Check sheet for the modelled part. Datum: model origin and axes. Units: mm. A direction names the side the tool comes from. Round coordinates to 2 decimals unless told otherwise and drop trailing zeros. Order: outer loops, then holes, each group sorted by start corner. A loop starts at its lowest first (then second) coordinate and runs counter-clockwise, first axis right, second up.
Q1. Cross-section at D-D on z = 5. Record the cut outline in (x, y).
Q2. Scan lines: probe 1 along Y at (x, z) = (21, 12.5); probe 2 along Y at (x, z) = (-26, 4.25); probe 3 along X at (y, z) = (21, 2). Record each from-to range of solid material in increasing order.
Q3. Cross-section at B-B on y = 32.5. Record the cut outline in (x, z), then the cut area to 3 significant figures.
Q4. Depth check by flat-ended pin: P1, Ø8, axis at x = 22, y = 21, coming from the +Z side; P2, Ø9, axis at y = 21.5, z = 12, coming from the +X side; P3, Ø2, axis at y = 36, z = 5, coming from the -X side. Enter the tip coordinate at first touch or a pass-through.
Q5. Mould release check, pull along X, two halves, no side actions. Record for faces 1 (the flat face through (0, 20, 4)), 2 (the flat face through (-1, 1, 14)): +X half, -X half, draft (parallel to the pull), parting line (faces both ways), or undercut.
Q6. Cross-section at A-A on x = -6.5. Record the cut outline in (y, z).
Q7. Cross-section at C-C on z = -4. Record the cut outline in (x, y).
Q8. Set-up check for faces 3 (the flat face through (-1, 38.11, 10)), 4 (the flat face through (-24, 34.688, 2)), 5 (the cylindrical face through (21.964, 19.72, 2.353)): record each of +Z, -Z, +X, -X, +Y, -Y from which the full face is reachable in a straight line by a thin tool's end or side.
from build123d import *

# Parameters (mm, degrees)
SKETCH1_R           = 2.5
BOSS_EXTRUDE2_DEPTH = 40
SKETCH3_W           = 90
SKETCH3_H           = 36.22
SKETCH3_R           = 1.5
SKETCH3_W_2         = 40
SKETCH3_H_2         = 2.46
CUT_EXTRUDE1_DEPTH  = 8
SKETCH3_5_W         = 40
SKETCH3_5_H         = 2.46
SKETCH3_5_R         = 1.5
CUT_EXTRUDE3_DEPTH  = 22.585745164


with BuildPart() as part:
    # Sketch1 → Boss-Extrude2 (new body)
    with BuildSketch(Plane(origin=(0, 0, 0), x_dir=(1, 0, 0), z_dir=(0, 1, 0))):
        with BuildLine():
            Line((-45, -14), (45, -14))
            ThreePointArc((45, -14), (47.968786967, -11.849318779), (49.443427998, -8.493047098))
            ThreePointArc((49.443427998, -8.493047098), (39.902505959, 6.907779255), (23.154454386, 0))
            ThreePointArc((23.154454386, 0), (21.939767311, -2.382145151), (19.810770857, -4))
            Line((19.810770857, -4), (-19.810770857, -4))
            ThreePointArc((-19.810770857, -4), (-21.939767311, -2.382145151), (-23.154454386, 0))
            ThreePointArc((-23.154454386, 0), (-39.902505959, 6.907779255), (-49.443427998, -8.493047098))
            ThreePointArc((-49.443427998, -8.493047098), (-47.968786967, -11.849318779), (-45, -14))
        make_face()
        with Locations((-42, 0)):
            Circle(SKETCH1_R, mode=Mode.SUBTRACT)
        with Locations((42, 0)):
            Circle(SKETCH1_R, mode=Mode.SUBTRACT)
    extrude(amount=BOSS_EXTRUDE2_DEPTH)

    # Sketch3 → Cut-Extrude1 (cut)
    with BuildSketch(Plane.XY.offset(14)):
        with Locations((0, 20)):
            Rectangle(SKETCH3_W, SKETCH3_H)
        with Locations((37.527569226, 35.802060635)):
            Circle(SKETCH3_R, mode=Mode.SUBTRACT)
        with Locations((-37.672430774, 35.802060635)):
            Circle(SKETCH3_R, mode=Mode.SUBTRACT)
        with Locations((-37.672430774, 4.382060635)):
            Circle(SKETCH3_R, mode=Mode.SUBTRACT)
        with Locations((37.527569226, 4.382060635)):
            Circle(SKETCH3_R, mode=Mode.SUBTRACT)
        with Locations((-15.072430774, 35.917939365)):
            Rectangle(SKETCH3_W_2, SKETCH3_H_2, mode=Mode.SUBTRACT)
    extrude(amount=-CUT_EXTRUDE1_DEPTH, mode=Mode.SUBTRACT)

    # Sketch3<5> → Cut-Extrude3 (cut, through all)
    with BuildSketch(Plane.XY.offset(14)):
        with Locations((-15.072430774, 35.917939365)):
            Rectangle(SKETCH3_5_W, SKETCH3_5_H)
        with Locations((-37.672430774, 35.802060635)):
            Circle(SKETCH3_5_R)
        with Locations((-37.672430774, 4.382060635)):
            Circle(SKETCH3_5_R)
        with Locations((37.527569226, 4.382060635)):
            Circle(SKETCH3_5_R)
        with Locations((37.527569226, 35.802060635)):
            Circle(SKETCH3_5_R)
    extrude(amount=-CUT_EXTRUDE3_DEPTH, mode=Mode.SUBTRACT)


solid = part.part
Results found:
1. outline: (-49.53, 0) - (49.53, 0) - (49.53, 40) - (-49.53, 40) - close; hole circle Ø3 at (-37.67, 4.38); hole circle Ø3 at (-37.67, 35.8); hole (-35.07, 34.69) - (4.93, 34.69) - (4.93, 37.15) - (-35.07, 37.15) - close; hole circle Ø3 at (37.53, 4.38); hole circle Ø3 at (37.53, 35.8)
2. probe 1: y = 0 to 1.89, 38.11 to 40
2. probe 2: y = 0 to 34.69, 37.15 to 40
2. probe 3: x = -48.88 to -43.5, -40.5 to -22.23, 22.23 to 40.5, 43.5 to 48.88
3. outline: (-49.44, 8.49) arc R14 ccw to (-23.15, 0) arc R6 cw to (-19.81, 4) - (19.81, 4) arc R6 cw to (23.15, 0) arc R14 ccw to (49.44, 8.49) arc R7 ccw to (45, 14) - (45, 6) - (-45, 6) - (-45, 14) arc R7 ccw to start; hole circle Ø5 at (-42, 0); hole circle Ø5 at (42, 0)
3. area: 699 mm2
4. P1: stops at z = 6
4. P2: stops at x = 49.56
4. P3: stops at x = -49.59
5. face 1: undercut
5. face 2: draft
6. outline: (0, 4) - (34.69, 4) - (34.69, 6) - (1.89, 6) - (1.89, 14) - (0, 14) - close; (37.15, 4) - (40, 4) - (40, 14) - (38.11, 14) - (38.11, 6) - (37.15, 6) - close
7. outline: (-44.96, 0) - (-26.24, 0) - (-26.24, 34.69) - (-35.07, 34.69) - (-35.07, 37.15) - (-26.24, 37.15) - (-26.24, 40) - (-44.96, 40) - close; (26.24, 0) - (44.96, 0) - (44.96, 40) - (26.24, 40) - close; hole circle Ø3 at (-37.67, 4.38); hole circle Ø3 at (-37.67, 35.8); hole circle Ø3 at (37.53, 4.38); hole circle Ø3 at (37.53, 35.8)
8. face 3: +Z
8. face 4: +Z, -Z
8. face 5: -Z, +Y, -Y
